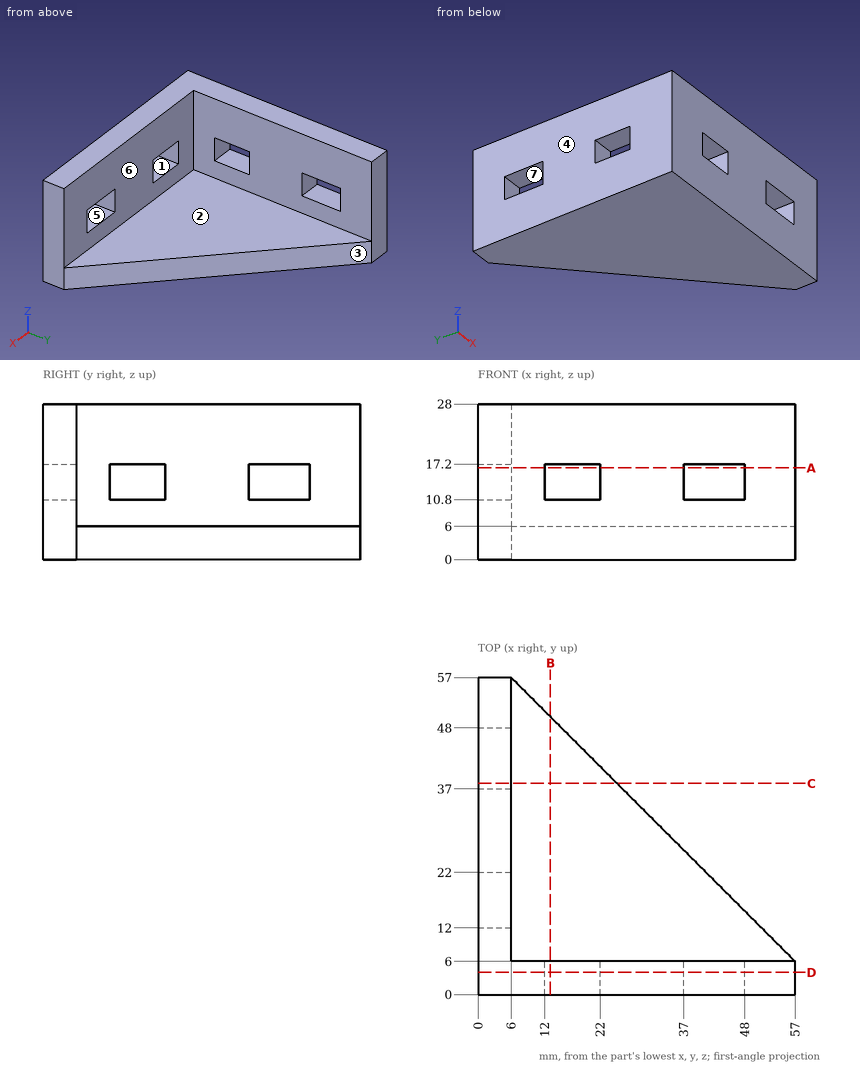
Input: dimensioned drawing with shaded views. Units: mm. Origin: part minimum x, y, z. A direction names the side the tool comes from. Give positions to 0.01 mm unless a question says otherwise; leave off trailing zeros. Loops run counter-clockwise (first coordinate to the right, second up) from the corner with the lowest first, then second, coordinate; pieces in that order, holes last. Notation, with made-up numbers: M 52.5,5 L 105.5,5 A32 cw 105.5,33 Z; hole C 25.5,78.25 d2. An arc over 180 degrees is marked long. Put each result on its own line as item: value.
1) Cut plane A-A, the plane z = 16.5. Return the cut outline in (x, y).
Computed values:
outline: M 0,0 L 12,0 L 12,6 L 6,6 L 6,12 L 0,12 Z; M 0,22 L 6,22 L 6,37 L 0,37 Z; M 0,48 L 6,48 L 6,57 L 0,57 Z; M 22,0 L 37,0 L 37,6 L 22,6 Z; M 48,0 L 57,0 L 57,6 L 48,6 Z
2) Reachability of the marked faces 5, 6 and 7 from +Z, -Z, +X, -X, +Y, -Y: full face, straight path, thin tool, end or side. Return the list, or none.
Computed values:
face 5: +Y, -Y
face 6: +Z, +X, +Y
face 7: +X, -X
3) First-contact query: P1, Ø12, axis at x = 13, y = 31.5, coming from the +Z side; P2, Ø8, axis at x = 29.5, z = 22.5, coming from the +Y side; P3, Ø6, axis at y = 29.5, z = 10.5, coming from the +X side. Flat tips, straight axial feed; report the tip coordinate or a pass-through.
Computed values:
P1: stops at z = 6
P2: stops at y = 6
P3: stops at x = 6
4) Cut plane D-D, the plane y = 4. Return the cut outline in (x, z), plus the area to 3 significant figures.
Computed values:
outline: M 0,0 L 57,0 L 57,28 L 0,28 Z; hole M 12,10.8 L 22,10.8 L 22,17.2 L 12,17.2 Z; hole M 37,10.8 L 48,10.8 L 48,17.2 L 37,17.2 Z
area: 1,460 mm^2
5) Material intervals for L1, parallel to Z at x = 4.5, y = 47.5; L2, parallel to Y at x = 54.5, z = 16.75, sorted ascending. Write a range as from..to.
Computed values:
L1: z = 0..10.8, 17.2..28
L2: y = 0..6
6) Cut plane C-C, the plane y = 38. Return the cut outline in (x, z).
Computed values:
outline: M 0,0 L 25,0 L 25,6 L 6,6 L 6,10.8 L 0,10.8 Z; M 0,17.2 L 6,17.2 L 6,28 L 0,28 Z
7) Mould query, pull axis X, two halves, no side actions, for the marked faces 1, 2, 3 and 4. Classes: released by +X, released by -X, zero draft, split by the parting line, or undercut.
Computed values:
face 1: undercut
face 2: zero draft
face 3: released by +X
face 4: released by -X
8) Cut plane B-B, the plane x = 13. Return the cut outline in (y, z).
Computed values:
outline: M 0,0 L 50,0 L 50,6 L 6,6 L 6,10.8 L 0,10.8 Z; M 0,17.2 L 6,17.2 L 6,28 L 0,28 Z
